Can you work these out from the model? Positions are in its coordinate system, mm. A direction names the side the tool comes from. Round coordinates to 2 decimals unless told otherwise and drop trailing zeros. Loops run counter-clockwise (first coordinate to the right, second up) from the corner with the lowest first, then second, coordinate; pieces in that order, holes last. Notation, with made-up numbers: (-19.5, -34.75) -> (5.5, -34.75) arc R24 ccw to (5.5, -16.75) -> close; hole circle Ø1 at (8, 49). An arc over 180 degrees is marked (long way). Answer as a JSON object with one key per item and string values.
```python
from build123d import *

# Parameters (mm, degrees)
SKETCH1_W           = 50
SKETCH1_H           = 6
BOSS_EXTRUDE1_DEPTH = 20
SKETCH2_R           = 3
CUT_EXTRUDE1_DEPTH  = 33.57299495
SKETCH3_W           = 135
SKETCH3_H           = 6
BOSS_EXTRUDE2_DEPTH = 40
SKETCH4_R           = 3
CUT_EXTRUDE2_DEPTH  = 82.2480769


with BuildPart() as part:
    # Sketch1 → Boss-Extrude1 (new body)
    with BuildSketch(Plane(origin=(0, 0, 0), x_dir=(1, 0, 0), z_dir=(0, 1, 0))):
        Rectangle(SKETCH1_W, SKETCH1_H)
    extrude(amount=BOSS_EXTRUDE1_DEPTH)

    # Sketch2 → Cut-Extrude1 (cut, through all)
    with BuildSketch(Plane(origin=(0, 0, -3), x_dir=(-1, 0, 0), z_dir=(0, 0, -1))):
        with Locations((-7.5, 15)):
            Circle(SKETCH2_R)
        with Locations((7.5, 15)):
            Circle(SKETCH2_R)
    extrude(amount=-CUT_EXTRUDE1_DEPTH, mode=Mode.SUBTRACT)

    # Sketch3 → Boss-Extrude2 (add)
    with BuildSketch(Plane(origin=(0, 0, -3), x_dir=(-1, 0, 0), z_dir=(0, 0, -1))):
        with Locations((0, 3)):
            Rectangle(SKETCH3_W, SKETCH3_H)
    extrude(amount=BOSS_EXTRUDE2_DEPTH)

    # Sketch4 → Cut-Extrude2 (cut, through all)
    with BuildSketch(Plane(origin=(0, 6, 0), x_dir=(1, 0, 0), z_dir=(0, 1, 0))):
        with Locations(Location((-57.5, 35, 0), (0, 0, 180))):
            Circle(SKETCH4_R)
        with Locations(Location((-42.5, 35, 0), (0, 0, 180))):
            Circle(SKETCH4_R)
        with Locations((42.5, 35)):
            Circle(SKETCH4_R)
        with Locations((57.5, 35)):
            Circle(SKETCH4_R)
    extrude(amount=-CUT_EXTRUDE2_DEPTH, mode=Mode.SUBTRACT)


solid = part.part
```
Q1. On a 3-axis mill with a long thin cutter (end or side, diameter ignored), from which of +Z, -Z, +X, -X, +Y, -Y can I reach the whole of each face in a straight line? I mean faces 4 (the flat face through (0, 13, -3)), 5 (the cylindrical face through (54.5, 3, -35.1)), 6 (the flat face through (47, 3, -3)), 7 (the flat face through (-25, 10, 0)), 8 (the flat face through (0, 10, 3)). Say none if no direction works.
Determined:
{"face 4": "-Z, +X, -X, +Y", "face 5": "+Y, -Y", "face 6": "+Z, +X, +Y, -Y", "face 7": "+Z, -X, +Y, -Y", "face 8": "+Z, +X, -X, +Y, -Y"}
Q2. If I drill on L1, parallel to Z at x = -57.5, y = 4.5; L2, parallel to Y at x = 7.5, z = -1; L3, parallel to X at y = 5, z = -34.5, over which ranges is the centre line in solid material (lowest first)? Write a range as [from, to].
Determined:
{"L1": "[-43, -38], [-32, -3]", "L2": "[0, 12], [18, 20]", "L3": "[-67.5, -60.46], [-54.54, -45.46], [-39.54, 39.54], [45.46, 54.54], [60.46, 67.5]"}
Q3. I want a section at C-C, the plane z = -35. Write out the boundary of the cut face in (x, y).
Determined:
{"outline": "(-67.5, 0) -> (-60.5, 0) -> (-60.5, 6) -> (-67.5, 6) -> close; (-54.5, 0) -> (-45.5, 0) -> (-45.5, 6) -> (-54.5, 6) -> close; (-39.5, 0) -> (39.5, 0) -> (39.5, 6) -> (-39.5, 6) -> close; (45.5, 0) -> (54.5, 0) -> (54.5, 6) -> (45.5, 6) -> close; (60.5, 0) -> (67.5, 0) -> (67.5, 6) -> (60.5, 6) -> close"}
Q4. I want a section at B-B, the plane x = -7.5. Write out the boundary of the cut face in (y, z).
Determined:
{"outline": "(0, -43) -> (6, -43) -> (6, -3) -> (12, -3) -> (12, 3) -> (0, 3) -> close; (18, -3) -> (20, -3) -> (20, 3) -> (18, 3) -> close"}
Q5. I want a section at D-D, the plane x = -57.5. Write out the boundary of the cut face in (y, z).
Determined:
{"outline": "(0, -43) -> (6, -43) -> (6, -38) -> (0, -38) -> close; (0, -32) -> (6, -32) -> (6, -3) -> (0, -3) -> close"}
Q6. We'd pull the mould along Y, two halves only. Please class faces 1 (the cylindrical face through (-8.884, 12.338, -0.042)), 2 (the flat face through (1, 6, -23)), 3 (the flat face through (-67.5, 3, -23)): pulls with the +Y half, pulls with the -Y half, needs draft (parallel to the pull), parting line crosses it, or undercut.
Determined:
{"face 1": "undercut", "face 2": "pulls with the +Y half", "face 3": "needs draft"}
Q7. I want a section at A-A, the plane y = 15. Write out the boundary of the cut face in (x, z).
Determined:
{"outline": "(-25, -3) -> (-10.5, -3) -> (-10.5, 3) -> (-25, 3) -> close; (-4.5, -3) -> (4.5, -3) -> (4.5, 3) -> (-4.5, 3) -> close; (10.5, -3) -> (25, -3) -> (25, 3) -> (10.5, 3) -> close"}
Q8. I'm going to push flat-ended pins straight in: pin 1 (12 mm diameter, centred on x = 27.5, z = -23, fed in from +Y); pin 2 (3.5 mm diameter, centred on x = 42.5, z = -35, fed in from -Y); pin 3 (5 mm diameter, centred on x = -38, y = 2.5, fed in from +Z); pin 4 (4 mm diameter, centred on x = -46, z = -26.5, fed in from -Y). Where does each tip first touch, or does it pass through?
Determined:
{"pin 1": "y = 6", "pin 2": "through", "pin 3": "z = -3", "pin 4": "y = 0"}
